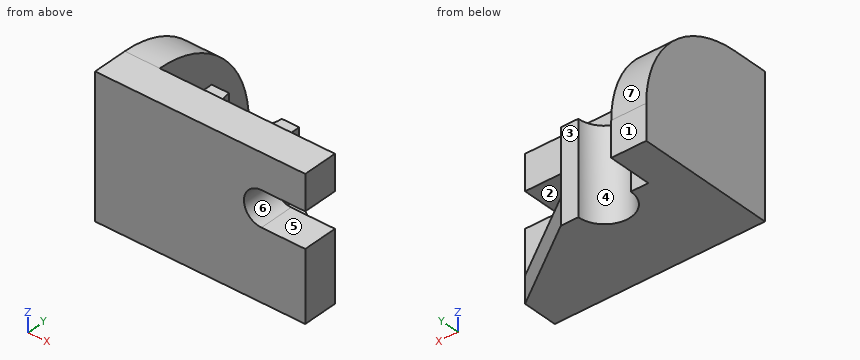
from build123d import *

# Parameters (mm, degrees)
SKETCH1_W           = 96
SKETCH1_H           = 64
BOSS_EXTRUDE1_DEPTH = 16
SKETCH2_W           = 16
SKETCH2_H           = 64
BOSS_EXTRUDE2_DEPTH = 48
FILLET3_R           = 48
SKETCH3_W           = 40
SKETCH3_H           = 42
BOSS_EXTRUDE3_DEPTH = 28
SKETCH4_R           = 12
CUT_EXTRUDE1_DEPTH  = 43
BOSS_EXTRUDE4_DEPTH = 12
CUT_EXTRUDE2_DEPTH  = 17


with BuildPart() as part:
    # Sketch1 → Boss-Extrude1 (new body)
    with BuildSketch(Plane(origin=(0, 0, 0), x_dir=(1, 0, 0), z_dir=(0, 1, 0))):
        Rectangle(SKETCH1_W, SKETCH1_H)
    extrude(amount=BOSS_EXTRUDE1_DEPTH)

    # Sketch2 → Boss-Extrude2 (add)
    with BuildSketch(Plane(origin=(0, 16, 0), x_dir=(1, 0, 0), z_dir=(0, 1, 0))):
        with Locations((-40, 0)):
            Rectangle(SKETCH2_W, SKETCH2_H)
    extrude(amount=BOSS_EXTRUDE2_DEPTH)

    # Fillet3
    fillet3_edges = [part.edges().sort_by_distance(p)[0] for p in [
        (-40, 64, 32),
    ]]
    fillet(fillet3_edges, radius=FILLET3_R)

    # Sketch3 → Boss-Extrude3 (add)
    with BuildSketch(Plane(origin=(0, 16, 0), x_dir=(1, 0, 0), z_dir=(0, 1, 0))):
        with Locations((-12, 11)):
            Rectangle(SKETCH3_W, SKETCH3_H)
    extrude(amount=BOSS_EXTRUDE3_DEPTH)

    # Sketch4 → Cut-Extrude1 (cut, through all)
    with BuildSketch(Plane.XY.offset(10)):
        with Locations((-12, 44)):
            Circle(SKETCH4_R)
    extrude(amount=-CUT_EXTRUDE1_DEPTH, mode=Mode.SUBTRACT)

    # Sketch5 → Boss-Extrude4 (add)
    with BuildSketch(Plane(origin=(0, 0, -32), x_dir=(-1, 0, 0), z_dir=(0, 0, -1))):
        Polygon((-8, 16), (-8, 44), (-48, 16), align=None)
    extrude(amount=-BOSS_EXTRUDE4_DEPTH)

    # Sketch6 → Cut-Extrude2 (cut, through all)
    with BuildSketch(Plane(origin=(0, 16, 0), x_dir=(1, 0, 0), z_dir=(0, 1, 0))):
        with BuildLine():
            Line((28, 0), (48, 0))
            ThreePointArc((48, 0), (56, -8), (48, -16))
            Line((48, -16), (28, -16))
            ThreePointArc((28, -16), (20, -8), (28, 0))
        make_face()
    extrude(amount=-CUT_EXTRUDE2_DEPTH, mode=Mode.SUBTRACT)


solid = part.part
Model file for the job. Use its own axes, mm. Face numbers are marked on the shaded views. A direction names the side the tool comes from. Round coordinates to 2 decimals unless told otherwise and drop trailing zeros. Loops run counter-clockwise (first coordinate to the right, second up) from the corner with the lowest first, then second, coordinate; pieces in that order, holes last. Notation, with made-up numbers: (-31, 63) - (25, 63) arc R19 ccw to (25, 100) - close; hole circle Ø5 at (56, -37.5). An arc over 180 degrees is marked (long way). Write each question's results on one line, items separated by ' | '.
(1) Saw through at B-B, the plane y = 36. List the corners of the cut face in (x, z).
Answer below:
outline: (-48, -32) - (-20.94, -32) - (-20.94, 10) - (-32, 10) - (-32, 27.63) - (-48, 27.63) - close; (-3.06, -32) - (19.43, -32) - (19.43, -20) - (8, -20) - (8, 10) - (-3.06, 10) - close
(2) 3-axis set-ups, long thin cutter, end or side, ignore diameter. For the marked faces 1, 2 and 3: which of +Z, -Z, +X, -X, +Y, -Y reach the whole face in a straight line?
Answer below:
face 1: +Z, -Z, +X, -X, +Y | face 2: +X, +Y, -Y | face 3: +Z, -Z, +X, +Y
(3) Pin check, flat tips, straight feed: pin 1 (6.5 mm diameter, centred on x = 5.5, z = -13, fed in from +Y); pin 2 (1 mm diameter, centred on x = 12, z = -12, fed in from +Y); pin 3 (2 mm diameter, centred on y = 41.5, z = -8.5, fed in from +X); pin 4 (10 mm diameter, centred on x = 0, y = 51.5, fed in from -Z). Stop position of each tip, or through.
Answer below:
pin 1: stops at y = 44 | pin 2: stops at y = 16 | pin 3: stops at x = 8 | pin 4: passes through
(4) Wall check: L1, parallel to Y at x = -5.5, z = 17; L2, parallel to Y at x = -12, z = -16.5; L3, parallel to X at y = 42.5, z = -10.5. Give the ranges that are in metal, low to high.
Answer below:
L1: y = 0 to 16 | L2: y = 0 to 32 | L3: x = -48 to -23.91, -0.09 to 8
(5) Saw through at C-C, the plane x = -38.5. List the corners of the cut face in (y, z).
Answer below:
outline: (0, -32) - (64, -32) - (64, -16) arc R48 ccw to (16, 32) - (0, 32) - close
(6) Saw through at D-D, the plane z = 8. List the corners of the cut face in (x, y).
Answer below:
outline: (-48, 0) - (20, 0) - (20, 16) - (8, 16) - (8, 44) - (0, 44) arc R12 cw to (-24, 44) - (-32, 44) - (-32, 57.57) - (-48, 57.57) - close
(7) Mould opens along Z. For the marked faces 4, 5, 6 and 7 say: released by +Z, released by -Z, zero draft, split by the parting line, or undercut.
Answer below:
face 4: zero draft | face 5: undercut | face 6: undercut | face 7: released by +Z
(8) Saw through at A-A, the plane y = 8.5. List the corners of the cut face in (x, z).
Answer below:
outline: (-48, -32) - (48, -32) - (48, 0) - (28, 0) arc R8 cw to (28, 16) - (48, 16) - (48, 32) - (-48, 32) - close
